Autodesk Inventor part; units mm, degrees
ref_plane "YZ Plane" through (0, 0, 0) normal (1, 0, 0) x (0, 1, 0)
ref_plane "XZ Plane" through (0, 0, 0) normal (0, 1, 0) x (-1, 0, 0)
ref_plane "XY Plane" through (0, 0, 0) normal (0, 0, 1) x (1, 0, 0)
sketch "Sketch1" plane through (0, 0, 0) normal (0, 1, 0) x (-1, 0, 0)
  circle A0 centre (0, 0) radius 2.4868
  line L0 (2.8868, 0) -> (1.4434, 2.5)
  line L1 (1.4434, 2.5) -> (-1.4434, 2.5)
  line L2 (-1.4434, 2.5) -> (-2.8868, 0)
  line L3 (-2.8868, 0) -> (-1.4434, -2.5)
  line L4 (-1.4434, -2.5) -> (1.4434, -2.5)
  line L5 (1.4434, -2.5) -> (2.8868, 0)
  line L6 (0, 0) -> (-23.467, 0)
  circle A1 centre (-49, 0) radius 2.4868
  line L7 (-46.1132, 0) -> (-47.5566, 2.5)
  line L8 (-47.5566, 2.5) -> (-50.4434, 2.5)
  line L9 (-50.4434, 2.5) -> (-51.8868, 0)
  line L10 (-51.8868, 0) -> (-50.4434, -2.5)
  line L11 (-50.4434, -2.5) -> (-47.5566, -2.5)
  line L12 (-47.5566, -2.5) -> (-46.1132, 0)
  arc A2 (43.788, 27) -> (35.788, 35) centre (35.788, 27) ccw
  line L13 (35.788, 35) -> (-48.212, 35)
  arc A3 (-48.212, 35) -> (-56.212, 27) centre (-48.212, 27) ccw
  line L14 (-56.212, 27) -> (-56.212, -62.0882)
  arc A4 (-56.212, -62.0882) -> (-54.3404, -67.2305) centre (-48.212, -62.0882) ccw
  line L15 (-54.3404, -67.2305) -> (-37.6324, -87.1423)
  arc A5 (-37.6324, -87.1423) -> (-31.504, -90) centre (-31.504, -82) ccw
  line L16 (-31.504, -90) -> (19.08, -90)
  arc A6 (19.08, -90) -> (25.2084, -87.1423) centre (19.08, -82) ccw
  line L17 (25.2084, -87.1423) -> (41.9164, -67.2305)
  arc A7 (41.9164, -67.2305) -> (43.788, -62.0882) centre (35.788, -62.0882) ccw
  line L18 (43.788, -62.0882) -> (43.788, 27)
  arc A8 (-17.212, -66) -> (-11.212, -72) centre (-11.212, -66) ccw
  line L19 (-11.212, -72) -> (-1.212, -72)
  arc A9 (-1.212, -72) -> (4.788, -66) centre (-1.212, -66) ccw
  line L20 (4.788, -66) -> (4.788, -64)
  arc A10 (10.788, -58) -> (4.788, -64) centre (10.788, -64) ccw
  line L21 (10.788, -58) -> (25.4731, -58)
  arc A11 (29.3447, -59.4162) -> (25.4731, -58) centre (25.4731, -64) ccw
  line L22 (29.3447, -59.4162) -> (31.3866, -61.1409)
  arc A12 (32.1113, -69.5814) -> (31.3866, -61.1409) centre (27.515, -65.7247) ccw
  line L23 (32.1113, -69.5814) -> (21.8111, -81.8567)
  arc A13 (17.2148, -84) -> (21.8111, -81.8567) centre (17.2148, -78) ccw
  line L24 (17.2148, -84) -> (-29.6388, -84)
  arc A14 (-34.2351, -81.8567) -> (-29.6388, -84) centre (-29.6388, -78) ccw
  line L25 (-34.2351, -81.8567) -> (-44.5353, -69.5814)
  arc A15 (-43.8106, -61.1409) -> (-44.5353, -69.5814) centre (-39.939, -65.7247) ccw
  line L26 (-43.8106, -61.1409) -> (-41.7687, -59.4162)
  arc A16 (-37.8971, -58) -> (-41.7687, -59.4162) centre (-37.8971, -64) ccw
  line L27 (-37.8971, -58) -> (-23.212, -58)
  arc A17 (-17.212, -64) -> (-23.212, -58) centre (-23.212, -64) ccw
  line L28 (-17.212, -64) -> (-17.212, -66)
  circle A18 centre (0, -58) radius 1.375
  circle A19 centre (0, 0) radius 1.5
  circle A20 centre (-49, -58) radius 1.375
  circle A21 centre (-51.962, 9) radius 0.575
  circle A22 centre (39.538, 27) radius 0.575
  circle A23 centre (39.538, 9) radius 0.575
  circle A24 centre (36.576, 0) radius 1.5
  circle A25 centre (36.576, -43.18) radius 1.5
  circle A26 centre (0, -43.18) radius 1.5
  circle A27 centre (-49, 0) radius 1.375
  circle A28 centre (-51.962, 27) radius 0.575
  circle A29 centre (-6.212, -53.538) radius 1.15
  circle A30 centre (-6.212, -67) radius 1.15
  line L29 (35.788, 35) -> (-48.212, 35)
  line L30 (-6.212, 35) -> (-6.212, -103.5846)
  dimension "d2" = 49
sketch "Sketch2" plane through (0, 0, 0) normal (0, 1, 0) x (-1, 0, 0)
  line L0 (-2.8868, 0) -> (-1.4434, -2.5)
  line L1 (1.4434, -2.5) -> (2.8868, 0)
  circle A0 centre (0, 0) radius 2.8868
  circle A1 centre (0, 0) radius 6
  arc A2 (0, -6) -> (0, -2.8868) centre (0, -4.4434) ccw
  arc A3 (0, 2.8868) -> (0, 6) centre (-0.1105, 4.4434) ccw
  line L2 (0, -4.4434) -> (-24.5, -4.4434)
  line L3 (-24.5, -4.4434) -> (-24.5, 4.4434)
  line L4 (-24.5, 4.4434) -> (0, 4.4434)
  line L5 (0, 4.4434) -> (0, -4.4434)
  line L6 (-46.1132, 0) -> (-47.5566, -2.5)
  line L7 (-50.4434, -2.5) -> (-51.8868, 0)
  circle A4 centre (-49, 0) radius 2.8868
  circle A5 centre (-49, 0) radius 6
  arc A6 (-49, -2.8868) -> (-49, -6) centre (-49, -4.4434) ccw
  arc A7 (-49, 6) -> (-49, 2.8868) centre (-48.8895, 4.4434) ccw
  line L8 (-49, -4.4434) -> (-24.5, -4.4434)
  line L9 (-24.5, 4.4434) -> (-49, 4.4434)
  line L10 (-49, 4.4434) -> (-49, -4.4434)
  circle A8 centre (-24.5, 0) radius 1.55
  line L11 (-6.212, 35) -> (-6.212, -103.5846)
  line L12 (0, 4.4434) -> (-12.424, 4.4434)
  line L13 (-12.424, 4.4434) -> (-12.424, 14.4434)
  line L14 (-12.424, 14.4434) -> (0, 14.4434)
  line L15 (0, 14.4434) -> (0, 4.4434)
  line L16 (-12.424, 4.4434) -> (-2.8868, 4.4434)
  line L17 (-2.8868, 4.4434) -> (-2.8868, 0)
  line L18 (-2.8868, 0) -> (-12.424, 0)
  line L19 (-12.424, 0) -> (-12.424, 4.4434)
  line L20 (-6.212, 4.4434) -> (-3.212, 4.4434)
  line L21 (-3.212, 4.4434) -> (-3.212, 12.4434)
  line L22 (-3.212, 12.4434) -> (-6.212, 12.4434)
  line L23 (-6.212, 12.4434) -> (-6.212, 4.4434)
  line L24 (-6.212, 4.4434) -> (-9.212, 4.4434)
  line L25 (-9.212, 4.4434) -> (-9.212, 12.4434)
  line L26 (-9.212, 12.4434) -> (-6.212, 12.4434)
  line L27 (-12.424, 4.4434) -> (-2.8868, 0)
  point P0 (0, 0)
  point P1 (-4.0319, -4.4434)
  point P2 (-4.0319, 4.4434)
  point P3 (-44.9681, 4.4434)
  point P4 (-44.9681, -4.4434)
  point P5 (0, 6)
  point P6 (0, 6)
  point P7 (-9.5372, 4.4434)
  point P8 (-3.212, 5.0678)
  dimension "d7" = 12
  dimension "d9" = 3.1
  dimension "d14" = 12.424
  dimension "d15" = 10
  dimension "d16" = 6.212
  dimension "d24" = 3
  dimension "d25" = 8
extrude "Extrusion1" add sketch "Sketch2" along normal blind 4 contours L17 L4 L5 A0 | L27 A1 L4 L17 | A0 L5 L2 A1 L18 | L18 A1 L27 | L5 L15 A3 | L4 L21 A1 L15 | L18 L11 L27 A1 | A1 L2 L11 L18 | L27 L11 L4 A1 | A2 A1 L2 L5 | L18 L19 L27 L11 | L11 L2 L3 A8 L4 L19 L18 | L27 L4 L11 | L8 A5 L9 L3 A8 | L8 L10 A4 L9 A5 | A5 A6 L10 L8 | L9 L10 A7 A5
extrude "Extrusion3" add sketch "Sketch2" along normal blind 10 contours L17 L4 L5 A0 | L27 A1 L4 L17 | L5 L15 A3 | L4 L21 A1 L15 | L27 L11 L4 A1 | A1 L21 L22 L11 L14 L15 | L27 L4 L11 | L13 L14 L11 L26 L25 L4
sketch "Sketch4" plane through (12.424, 0, 14.4434) normal (1, 0, 0) x (0, 0, -1)
  line L0 (2, 0) -> (2, 10)
  line L1 (2, 10) -> (10, 10)
  line L2 (10, 10) -> (10, 0)
  line L3 (10, 0) -> (2, 0)
  line L4 (2, 0) -> (2, 10)
  circle A0 centre (5, 6) radius 1.55
  point P0 (14.4434, 0)
  dimension "d26" = 8
  dimension "d27" = 3.1
  dimension "d28" = 4
  dimension "d31" = 3
extrude "Extrusion4" cut sketch "Sketch4" against normal up to surface (12.424 mm away) contours A0
fillet "Fillet3" radius 3 2 edges at (7.6554, 4, 2.2217) (7.6554, 10, 2.2217)
fillet "Fillet3" radius 2 7 edges at (12.424, 2, 4.4434) (12.424, 5, 14.4434) (0, 5, 14.4434) (44.9681, 2, 4.4434) (44.9681, 2, -4.4434) (4.0319, 2, -4.4434) (0, 5, 6)
equation "\"d14\" = 2 * d16"
equation "\"d24\" = Acrylic"
equation "\"Acrylic\" = 3"
properties part number "BaseMount"
The listing builds one solid part. Answer for the finished solid, in the listing's coordinates (mm). A direction names the side the tool comes from. Coordinates: 2 decimals unless noted, no trailing zeros. Write each loop counter-clockwise with the first axis right and the second up, starting at its lowest first coordinate (ties: lowest second). Pieces come first, ordered by that corner, then holes.
Q1. The mould has two halves that part along Z. Classify faces 5 (the cylindrical face through (47.1, 1.97, -5.69)), 6 (the flat face through (19, 0, 2)), 7 (the flat face through (9.212, 5, 7)), 8 (the flat face through (6, 5, 4.443)): released by +Z, released by -Z, zero draft, split by the parting line, or undercut.
Returned:
face 5: released by -Z
face 6: zero draft
face 7: undercut
face 8: undercut
Q2. Section B-B, the plane y = 6 is taken. Write down the section's boundary in (x, z).
Returned:
outline: (-0.81, 5.7) arc R1.56 ccw to (0, 2.89) arc R2.89 cw to (2.88, -0.19) - (13.42, 4.72) arc R2 cw to (12.42, 6.44) - (12.42, 7.89) - (9.21, 7.89) - (9.21, 4.44) - (3.21, 4.44) - (3.21, 7.89) - (0, 7.89) - (0, 7.31) arc R2 cw to start; (0, 10.99) - (3.21, 10.99) - (3.21, 12.44) - (9.21, 12.44) - (9.21, 10.99) - (12.42, 10.99) - (12.42, 12.44) arc R2 ccw to (10.42, 14.44) - (2, 14.44) arc R2 ccw to (0, 12.44) - close
Q3. Section D-D, the plane x = 32 is taken. Write down the section's boundary in (y, z), then the cut area to 3 significant figures.
Returned:
outline: (0, -4.44) - (4, -4.44) - (4, 4.44) - (0, 4.44) - close
area: 35.5 mm2
Q4. Find the intervals of material crossed by line 1 along X through (y, z) = (4, 8.75); line 2 along X through (y, z) = (1.25, 0); line 3 along Y through (x, z) = (14.5, 1.5), in increasing order.
Returned:
line 1: x = 0 to 3.21, 9.21 to 12.42
line 2: x = 2.89 to 22.95, 26.05 to 46.11
line 3: y = 0 to 4
Q5. Which of the six approach directions +Z, -Z, +X, -X, +Y, -Y give full straight-line access (tool end or side, diameter ignored) to faces 1 (the cylindrical face through (44.891, 1.972, -4.546)), 2 (the flat face through (31, 4, 0)), 3 (the flat face through (3.212, 5, 7)), 4 (the cylindrical face through (47.154, 1.972, 5.709))?
Returned:
face 1: -Z, +Y, -Y
face 2: -Z, +X, +Y
face 3: +Y, -Y
face 4: +Z, +Y, -Y
Q6. Section A-A, the plane x = 24.5 is taken. Write down the section's boundary in (y, z).
Returned:
outline: (0, -4.44) - (4, -4.44) - (4, -1.55) - (0, -1.55) - close; (0, 1.55) - (4, 1.55) - (4, 4.44) - (0, 4.44) - close
Q7. Given P1, Ø5.5, axis at y = 4, z = 9, coming from the -X side; P2, Ø6, axis at x = 24, z = 6, coming from the -Y side; P3, Ø1, axis at x = 34.5, z = 6.5, coming from the +Y side; P4, Ø5.5, axis at x = 29.5, y = 3, coming from the +Z side, each flat-ended and moving along its own axis, determine where each tip first touches the part or whether it passes through.
Returned:
P1: stops at x = -0.3
P2: stops at y = 0
P3: passes through
P4: stops at z = 4.44
Q8. Section C-C, the plane y = 9 is taken. Write down the section's boundary in (x, z).
Returned:
outline: (-0.81, 5.7) arc R1.56 ccw to (0, 2.89) arc R2.89 cw to (2.78, 0.79) - (12.71, 5.42) arc R2 cw to (12.42, 6.44) - (12.42, 12.44) arc R2 ccw to (10.42, 14.44) - (2, 14.44) arc R2 ccw to (0, 12.44) - (0, 7.31) arc R2 cw to start; hole (3.21, 4.44) - (9.21, 4.44) - (9.21, 12.44) - (3.21, 12.44) - close
